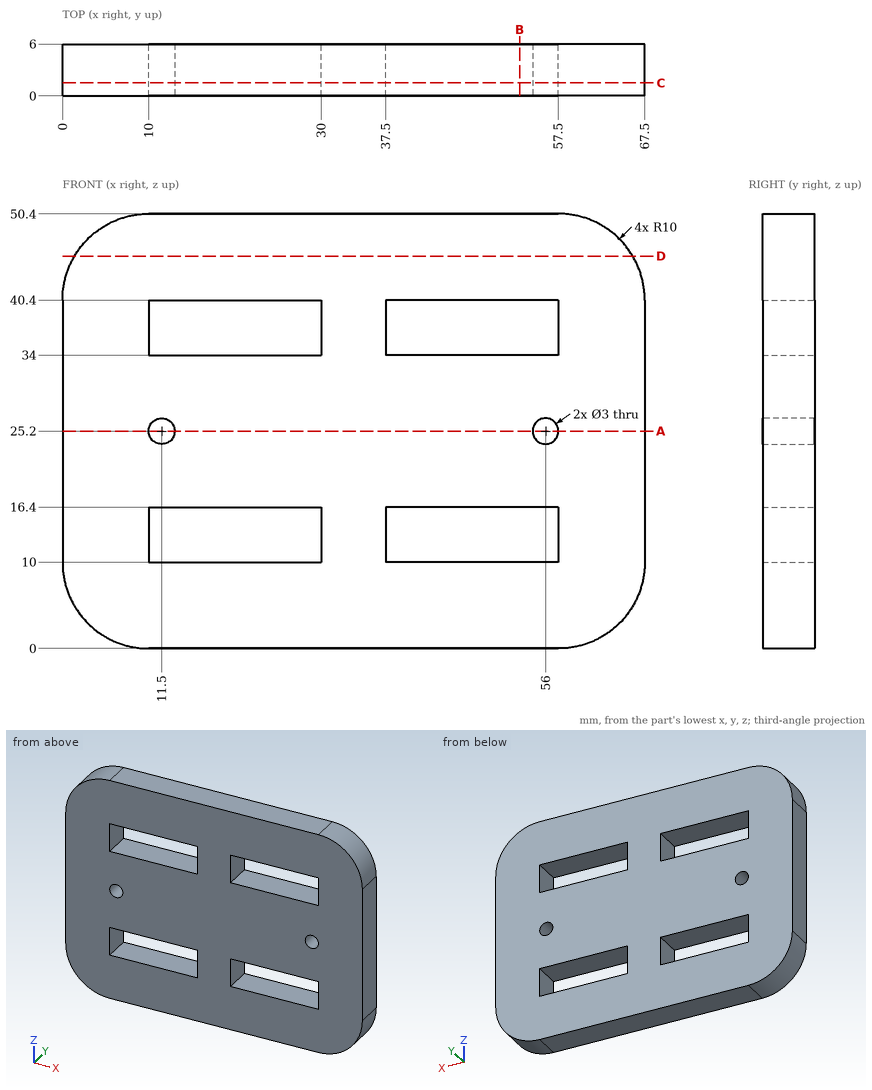
Job drawing, mm, ordinate dimensions from the low corner. One solid piece. Give positions to 0.01 mm unless a question says otherwise; leave off trailing zeros. Order: outer loops, then holes, each group sorted by start corner. A loop starts at its lowest first (then second) coordinate and runs counter-clockwise, first axis right, second up. Notation, with made-up numbers: M 14,-36 L 61,-36 A6 ccw 61,-30 Z; hole C -25.5,40.5 d7. An arc over 180 degrees is marked long. Return JSON: item names as keys, results as strings.
Q1. Band-saw the part on B-B (x = 53). Give the cut face in (y, z), then the cut area to 3 significant figures.
Answer list:
{"outline": "M 0,0 L 6,0 L 6,10 L 0,10 Z; M 0,16.4 L 6,16.4 L 6,34 L 0,34 Z; M 0,40.4 L 6,40.4 L 6,50.4 L 0,50.4 Z", "area": "226 mm^2"}
Q2. Band-saw the part on C-C (y = 1.5). Give the cut face in (x, z).
Answer list:
{"outline": "M 0,10 A10 ccw 10,0 L 57.5,0 A10 ccw 67.5,10 L 67.5,40.4 A10 ccw 57.5,50.4 L 10,50.4 A10 ccw 0,40.4 Z; hole M 10,10 L 30,10 L 30,16.4 L 10,16.4 Z; hole C 11.5,25.2 d3; hole M 10,34 L 30,34 L 30,40.4 L 10,40.4 Z; hole M 37.5,10 L 57.5,10 L 57.5,16.4 L 37.5,16.4 Z; hole M 37.5,34 L 57.5,34 L 57.5,40.4 L 37.5,40.4 Z; hole C 56,25.2 d3"}
Q3. Wall check: probe 1 along X at (y, z) = (4.3, 38); probe 2 along X at (y, z) = (4.6, 25.2); probe 3 along Z at (x, y) = (11.5, 4.2). Give the ranges that are in metal, low to high. Write a range as from..to.
Answer list:
{"probe 1": "x = 0..10, 30..37.5, 57.5..67.5", "probe 2": "x = 0..10, 13..54.5, 57.5..67.5", "probe 3": "z = 0..10, 16.4..23.7, 26.7..34, 40.4..50.4"}
Q4. Band-saw the part on A-A (z = 25.2). Give the cut face in (x, y), then the cut area to 3 significant figures.
Answer list:
{"outline": "M 0,0 L 10,0 L 10,6 L 0,6 Z; M 13,0 L 54.5,0 L 54.5,6 L 13,6 Z; M 57.5,0 L 67.5,0 L 67.5,6 L 57.5,6 Z", "area": "369 mm^2"}
Q5. Band-saw the part on D-D (z = 45.5). Give the cut face in (x, y).
Answer list:
{"outline": "M 1.4,0 L 66.1,0 L 66.1,6 L 1.4,6 Z"}
